```python
from build123d import *

# Parameters (mm, degrees)
SKETCH1_W                      = 228.6
SKETCH1_H                      = 25.4
BOSS_EXTRUDE1_DEPTH            = 25.4
SKETCH2_W                      = 22.225
SKETCH2_H                      = 22.225
CUT_EXTRUDE1_DEPTH             = 252.44717139
F_7_0_201_DIAMETER_HOLE1_D     = 5.1054
F_7_0_201_DIAMETER_HOLE1_DEPTH = 25.4
F_7_0_201_DIAMETER_HOLE2_D     = 5.1054


with BuildPart() as part:
    # Sketch1 → Boss-Extrude1 (new body)
    with BuildSketch(Plane(origin=(0, 101.6, 0), x_dir=(1, 0, 0), z_dir=(0, 1, 0))):
        with Locations((114.3, -12.7)):
            Rectangle(SKETCH1_W, SKETCH1_H)
    extrude(amount=-BOSS_EXTRUDE1_DEPTH)

    # Sketch2 → Cut-Extrude1 (cut, through all)
    with BuildSketch(Plane(origin=(228.6, 0, 0), x_dir=(0, 0, -1), z_dir=(1, 0, 0))):
        with Locations((-14.2875, 90.4875)):
            Rectangle(SKETCH2_W, SKETCH2_H)
    extrude(amount=-CUT_EXTRUDE1_DEPTH, mode=Mode.SUBTRACT)

    # #7 (0.201) Diameter Hole1
    with Locations(Plane.XZ.offset(-76.2)):
        with Locations((-12.7, -12.7), (38.1, 12.7), (63.5, 12.7), (88.9, 12.7), (114.3, 12.7), (139.7, 12.7), (165.1, 12.7), (190.5, 12.7), (215.9, 12.7)):
            Hole(F_7_0_201_DIAMETER_HOLE1_D / 2, depth=F_7_0_201_DIAMETER_HOLE1_DEPTH)

    # #7 (0.201) Diameter Hole2 (through all)
    with Locations(Plane.XY.offset(3.175)):
        with Locations((12.7, 88.9), (38.1, 88.9), (63.5, 88.9), (88.9, 88.9), (114.3, 88.9), (139.7, 88.9), (165.1, 88.9), (190.5, 88.9), (215.9, 88.9)):
            Hole(F_7_0_201_DIAMETER_HOLE2_D / 2)


solid = part.part
```
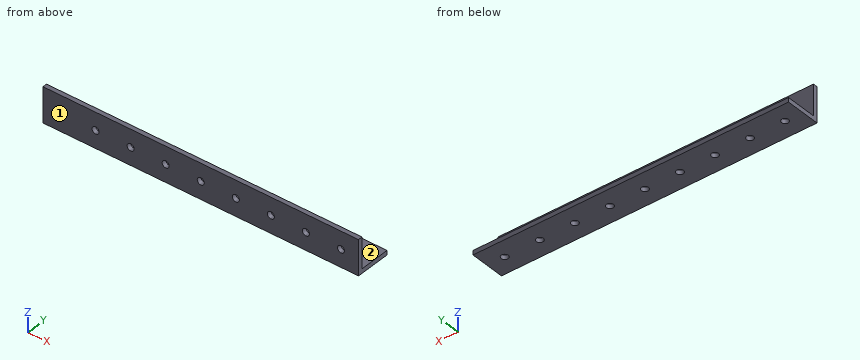
For this review, take the finished solid that the model builds, in its own axes (mm). Face numbers are marked on the shaded views. A direction names the side the tool comes from. Coordinates: 2 decimals unless noted, no trailing zeros. Loops run counter-clockwise (first coordinate to the right, second up) from the corner with the lowest first, then second, coordinate; pieces in that order, holes last.
1. Add section D-D, the plane x = 130.5. Give the boundary of the cut face in (y, z) (3 decimals), then the cut area to 3 significant figures.
2. For the marked faces 1 and 2, list the 3-axis set-ups (+Z, -Z, +X, -X, +Y, -Y) from which the entire face can be reached by the end or side of a thin tool; tool diameter is ignored.
3. Add section B-B, the plane z = 12.7. Count the separate pieces of the cut face and the enclosed holes in it, then the cut area to 3 significant figures.
4. For line 1 (Z direction, x = 38.1, y = 77.75); line 2 (Z direction, x = 148, y = 93.25) (3 decimals); line 3 (Y direction, x = 165.1, z = 1), list the stretches that pass through material, from the lowest coordinate up.
5. Add section C-C, the plane y = 83. Give the boundary of the cut face in (x, z) (3 decimals), then the cut area to 3 significant figures.
6. Add section A-A, the plane x = 88.9. Give the boundary of the cut face in (y, z) (3 decimals), then the cut area to 3 significant figures.
7. Insertion check: P1, Ø10, axis at x = 162, z = 4, coming from the +Y side; P2, Ø3, axis at x = 190.5, y = 88.9, coming from the -Z side; P3, Ø4, axis at x = 93, z = 12.5, coming from the +Y side (3 decimals); P4, Ø12, axis at x = 183.5, y = 98.5, coming from the +Z side (3 decimals). Each pin has a flat end and moves straight along its axis. Give the tip position at first contact, or say it passes through.
Result:
1. outline: (76.2, 0) - (101.6, 0) - (101.6, 3.175) - (79.375, 3.175) - (79.375, 25.4) - (76.2, 25.4) - close
1. area: 151 mm2
2. face 1: +Z, -Z, +X, -X, -Y
2. face 2: +Z, +X, -X, +Y
3. separate pieces: 9
3. enclosed holes: 0
3. area: 596 mm2
4. line 1: z = 0 to 10.15, 15.25 to 25.4
4. line 2: z = 0 to 3.175
4. line 3: y = 76.2 to 86.35, 91.45 to 101.6
5. outline: (0, 0) - (228.6, 0) - (228.6, 3.175) - (0, 3.175) - close
5. area: 726 mm2
6. outline: (76.2, 0) - (86.347, 0) - (86.347, 3.175) - (79.375, 3.175) - (79.375, 10.147) - (76.2, 10.147) - close; (76.2, 15.253) - (79.375, 15.253) - (79.375, 25.4) - (76.2, 25.4) - close; (91.453, 0) - (101.6, 0) - (101.6, 3.175) - (91.453, 3.175) - close
6. area: 119 mm2
7. P1: stops at y = 101.6
7. P2: passes through
7. P3: stops at y = 79.375
7. P4: stops at z = 3.175
